Verification items for the finished model (mm, model axes). Round coordinates to 2 decimals unless told otherwise and drop trailing zeros. Loops run counter-clockwise (first coordinate to the right, second up) from the corner with the lowest first, then second, coordinate; pieces in that order, holes last. Notation, with made-up numbers: M -37.5,34.5 L 10.5,34.5 A7 ccw 10.5,42.5 Z; hole C -31.75,70 d9. An arc over 180 degrees is marked long. Answer as CSV lines item,"result".
```python
from build123d import *

# Parameters (mm, degrees)
F5_DEPTH = 20
F6_DEPTH = 20


# Not quite as in the source:
# - the program builds the solid bodies; features that only make, move or delete a surface that nothing else refers to are left out


with BuildPart() as f5:
    # F4 (on offset) → F5 (new body)
    with BuildSketch(Plane.XY.offset(720)):
        with BuildLine():
            ThreePointArc((0, -260), (76.1522368915, -76.1522368915), (260, 0))
            Line((260, 0), (1035, 0))
            Line((1035, 0), (1035, 760))
            Line((1035, 760), (-575, 760))
            Line((-575, 760), (-575, -420))
            Line((-575, -420), (0, -420))
            Line((0, -420), (0, -260))
        make_face()
    extrude(amount=F5_DEPTH)

    # F4 (on offset) → F6 (join)
    with BuildSketch(Plane.XY.offset(720)):
        with BuildLine():
            ThreePointArc((0, -260), (76.1522368915, -76.1522368915), (260, 0))
            Line((260, 0), (1035, 0))
            Line((1035, 0), (1035, 760))
            Line((1035, 760), (-575, 760))
            Line((-575, 760), (-575, -420))
            Line((-575, -420), (0, -420))
            Line((0, -420), (0, -260))
        make_face()
        Polygon((0, -1240), (0, -420), (-575, -420), (-575, 760), (-760, 760), (-760, -1240), align=None)
    extrude(amount=-F6_DEPTH)


solid = f5.part
```
1) Section check B-B (x = -122). Record the cut outline in (y, z).
Here are the results:
outline,"M -1240,700 L 760,700 L 760,740 L -420,740 L -420,720 L -1240,720 Z"
2) Section check A-A (z = 709). Record the cut outline in (x, y), plus the area to 3 significant figures.
Here are the results:
outline,"M -760,-1240 L 0,-1240 L 0,-260 A260 cw 260,0 L 1035,0 L 1035,760 L -760,760 Z"
area,"2,320,000 mm^2"
3) Material ranges on probe 1 along Y at (x, z) = (898.5, 721); probe 2 along Z at (x, y) = (-283, -614); probe 3 along X at (y, z) = (-816, 704), recorded low to high.
Here are the results:
probe 1,"y = 0 to 760"
probe 2,"z = 700 to 720"
probe 3,"x = -760 to 0"
4) Go/stop test with flat-tipped pins: pin 1 (5 mm diameter, centred on x = 202, z = 731.5, fed in from -Y); pin 2 (6 mm diameter, centred on x = 71.5, z = 711.5, fed in from -Y); pin 3 (16 mm diameter, centred on y = 189.5, z = 734, fed in from -X). Record where each tip stops, or that it passes through.
Here are the results:
pin 1,"stops at y = -7.14"
pin 2,"stops at y = -84.14"
pin 3,"stops at x = -575"
5) Section check D-D (y = -879). Record the cut outline in (x, z).
Here are the results:
outline,"M -760,700 L 0,700 L 0,720 L -760,720 Z"
6) Section check C-C (y = 277). Record the cut outline in (x, z).
Here are the results:
outline,"M -760,700 L 1035,700 L 1035,740 L -575,740 L -575,720 L -760,720 Z"
